The listing builds one solid part. Answer for the finished solid, in the listing's coordinates (mm). A direction names the side the tool comes from. Give positions to 0.01 mm unless a question says otherwise; leave off trailing zeros. Write item = value, one per line. Start each with the question number.
1) Consider probe 1 along X at (y, z) = (4, -10); probe 2 along Z at (x, y) = (40, 13); probe 3 along Y at (x, z) = (-45.5, -20). Determine where each line is inside the solid, lowest interval first.
2) The part is cut by section A-A on y = 21. State how many separate pieces and enclosed holes the cut face has, plus the area to 3 significant figures.
3) Which of the six approach directions +Z, -Z, +X, -X, +Y, -Y give full straight-line access (tool end or side, diameter ignored) to faces 4 (the flat face through (7.503, 21, -50)), 5 (the flat face through (1, 0, -1)), 6 (the flat face through (1, 28, -48.5))?
4) The mould has two halves that part along X. Classify faces 1 (the flat face through (-52, 26, 1)), 2 (the flat face through (-7.497, 21, -50)), 3 (the flat face through (-1, 26, -52)): +X half, -X half, draft (parallel to the pull), parting line (faces both ways), or undercut.
5) Flat-ended cylindrical pins translate along their axes: P1, Ø10, axis at x = -36.5, y = 44, coming from the +Z side; P2, Ø1.8, axis at y = 30, z = -51, coming from the -X side; P3, Ø0.6, axis at y = 32.5, z = 50.5, coming from the +X side. Find the tip coordinate at first contact, or state that the pin passes through.
from build123d import *

# Parameters (mm, degrees)
SCHIZZO1_W                   = 100
SCHIZZO1_H                   = 100
ESTRUSIONE_ESTRUSIONE1_DEPTH = 2
ESTRUSIONE_ESTRUSIONE2_DEPTH = 52
ESTRUSIONE_ESTRUSIONE3_DEPTH = 54
RACCORDO1_R                  = 1
RACCORDO2_R                  = 1
RACCORDO3_R                  = 2
RACCORDO4_R                  = 2
RACCORDO5_R                  = 1
SCHIZZO4_R                   = 2.5
SCHIZZO4_W                   = 15.002685422
SCHIZZO4_H                   = 6.74925895
SCHIZZO4_W_2                 = 15
SCHIZZO4_H_2                 = 9
TAGLIO_ESTRUSIONE1_DEPTH     = 10


with BuildPart() as part:
    # Schizzo1 → Estrusione-Estrusione1 (new body)
    with BuildSketch(Plane(origin=(0, 0, 0), x_dir=(1, 0, 0), z_dir=(0, 1, 0))):
        Rectangle(SCHIZZO1_W, SCHIZZO1_H)
    extrude(amount=ESTRUSIONE_ESTRUSIONE1_DEPTH)

    # Schizzo2 → Estrusione-Estrusione2 (add)
    with BuildSketch(Plane(origin=(0, 0, 0), x_dir=(1, 0, 0), z_dir=(0, 1, 0))):
        Polygon((-50, -50), (-50, -52), (-52, -52), (-52, 52), (52, 52), (52, -52), (49.997213979, -52), (49.997213979, -50), (50, 50), (-50, 50), align=None)
    extrude(amount=ESTRUSIONE_ESTRUSIONE2_DEPTH)

    # Schizzo3 → Estrusione-Estrusione3 (add)
    with BuildSketch(Plane(origin=(0, 0, 0), x_dir=(1, 0, 0), z_dir=(0, 1, 0))):
        Polygon((-50, -50), (-50, 50), (50, 50), (49.997213979, -50), (48.497213979, -50), (48.497213979, 48.5), (-48.502786021, 48.5), (-48.502786021, -50), align=None)
    extrude(amount=ESTRUSIONE_ESTRUSIONE3_DEPTH)

    # Raccordo1
    raccordo1_edges = [part.edges().sort_by_distance(p)[0] for p in [
        (49.998606989, 54, 0),
        (0, 54, -50),
        (-50, 54, 0),
    ]]
    fillet(raccordo1_edges, radius=RACCORDO1_R)

    # Raccordo2
    raccordo2_edges = [part.edges().sort_by_distance(p)[0] for p in [
        (-50, 52, 0),
        (0, 52, -50),
    ]]
    fillet(raccordo2_edges, radius=RACCORDO2_R - 0.0001)  # a hair under: the kernel refuses the full size

    # Raccordo3
    raccordo3_edges = [part.edges().sort_by_distance(p)[0] for p in [
        (52, 26, 52),
        (52, 26, -52),
        (-52, 26, 52),
    ]]
    fillet(raccordo3_edges, radius=RACCORDO3_R - 0.0001)  # a hair under: the kernel refuses the full size

    # Raccordo4
    raccordo4_edges = [part.edges().sort_by_distance(p)[0] for p in [
        (-52, 26, -52),
    ]]
    fillet(raccordo4_edges, radius=RACCORDO4_R)

    # Raccordo5
    raccordo5_edges = [part.edges().sort_by_distance(p)[0] for p in [
        (5e-05, 0, -52),
        (52, 0, 0),
        (-51.414242852, 0, 51.414242852),
        (51.414242852, 0, 51.414242852),
        (51.414242852, 0, -51.414242852),
        (-52, 0, 5e-05),
        (-51.414213562, 0, -51.414213562),
        (49.998656989, 0, 52),
    ]]
    fillet(raccordo5_edges, radius=RACCORDO5_R)

    # Schizzo4 → Taglio-Estrusione1 (cut)
    with BuildSketch(Plane(origin=(0, 0, -52), x_dir=(-1, 0, 0), z_dir=(0, 0, -1))):
        with Locations((15, 21)):
            Circle(SCHIZZO4_R)
        with Locations((30.001342711, 21)):
            Circle(SCHIZZO4_R)
        with Locations((22.501342711, 31)):
            Rectangle(SCHIZZO4_W, SCHIZZO4_H)
        with Locations((-0.00336937, 21)):
            Rectangle(SCHIZZO4_W_2, SCHIZZO4_H_2)
    extrude(amount=-TAGLIO_ESTRUSIONE1_DEPTH, mode=Mode.SUBTRACT)


solid = part.part
Answer below:
q1.probe_1 = -52 to -48.5, 48.5 to 52
q1.probe_2 = -52 to -48.5
q1.probe_3 = 0 to 2
q2.separate_pieces = 4
q2.enclosed_holes = 0
q2.area = 971 mm2
q3.face_4 = +Z, -Z
q3.face_5 = +Z, -Z, +X, -X, -Y
q3.face_6 = +Z, +Y
q4.face_1 = -X half
q4.face_2 = undercut
q4.face_3 = draft
q5.P1 = -48.5
q5.P2 = -52
q5.P3 = 51.99
